Work out the finished part from the listing and answer in its coordinate system (mm). Round coordinates to 2 decimals unless told otherwise and drop trailing zeros. Loops run counter-clockwise (first coordinate to the right, second up) from the corner with the lowest first, then second, coordinate; pieces in that order, holes last. Notation, with made-up numbers: (44, 48) -> (89, 48) arc R16 ccw to (89, 68) -> close; hole circle Ø9 at (24, 72). An arc over 180 degrees is marked (long way). Write item = value, one per line. Start each with the question number.
```python
from build123d import *

# Parameters (mm, degrees)
BOSS_EXTRUDE1_DEPTH = 3


with BuildPart() as part:
    # Sketch1 → Boss-Extrude1 (new body)
    with BuildSketch(Plane.XY):
        with BuildLine():
            Line((711.17673453, 385), (499.657382069, 385))
            ThreePointArc((499.657382069, 385), (490.09029626, 383.096988313), (481.979712539, 377.67766953))
            Line((481.979712539, 377.67766953), (398.788878519, 294.486835509))
            ThreePointArc((398.788878519, 294.486835509), (393.369559736, 286.376251789), (391.466548048, 276.80916598))
            Line((391.466548048, 276.80916598), (391.466548048, 55))
            ThreePointArc((391.466548048, 55), (398.788878519, 37.32233047), (416.466548048, 30))
            Line((416.466548048, 30), (711.17673453, 30))
            ThreePointArc((711.17673453, 30), (728.85440406, 37.32233047), (736.17673453, 55))
            Line((736.17673453, 55), (736.17673453, 360))
            ThreePointArc((736.17673453, 360), (728.85440406, 377.67766953), (711.17673453, 385))
        make_face()
        Polygon((416.466548048, 276.80916598), (499.657382069, 360), (711.17673453, 360), (711.17673453, 276.80916598), align=None, mode=Mode.SUBTRACT)
    extrude(amount=-BOSS_EXTRUDE1_DEPTH)


solid = part.part
```
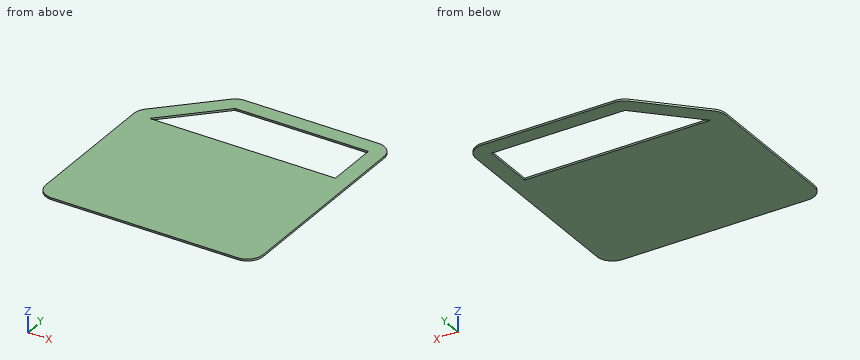
Item 1: Find the intervals of material crossed by line 1 along Y through (x, z) = (643, -0.8); line 2 along Y through (x, z) = (489, -1.8); line 3 along X through (y, z) = (331, -0.4), in increasing order. Write a range as [from, to].
Item 2: Section A-A (x = 507.5) is taken. Determine the outline of the cut face in (y, z), then the cut area to 3 significant figures.
Item 3: Section C-C (y = 348) is taken. Determine the outline of the cut face in (x, z), then the cut area to 3 significant figures.
Item 4: Section B-B (z = -0.6) is taken. Determine the outline of the cut face in (x, y).
Worked answers:
q1.line_1 = [30, 276.81], [360, 385]
q1.line_2 = [30, 276.81], [349.34, 382.61]
q1.line_3 = [435.3, 470.66], [711.18, 736.18]
q2.outline = (30, -3) -> (276.81, -3) -> (276.81, 0) -> (30, 0) -> close; (360, -3) -> (385, -3) -> (385, 0) -> (360, 0) -> close
q2.area = 815 mm2
q3.outline = (452.3, -3) -> (487.66, -3) -> (487.66, 0) -> (452.3, 0) -> close; (711.18, -3) -> (736.18, -3) -> (736.18, 0) -> (711.18, 0) -> close
q3.area = 181 mm2
q4.outline = (391.47, 55) arc R25 ccw to (416.47, 30) -> (711.18, 30) arc R25 ccw to (736.18, 55) -> (736.18, 360) arc R25 ccw to (711.18, 385) -> (499.66, 385) arc R25 ccw to (481.98, 377.68) -> (398.79, 294.49) arc R25 ccw to (391.47, 276.81) -> close; hole (416.47, 276.81) -> (711.18, 276.81) -> (711.18, 360) -> (499.66, 360) -> close
